Read the model definition and answer for the solid it produces. Units are mm, in the model's axes. Face numbers are marked on the shaded views. A direction names the side the tool comes from. Coordinates: 2 decimals unless noted, no trailing zeros. Write each loop counter-clockwise with the first axis right and the second up, starting at its lowest first coordinate (ties: lowest second). Pieces come first, ordered by that corner, then holes. Notation, with made-up numbers: (43, -38) -> (88, -38) arc R26 ccw to (88, -12) -> close; hole circle Ø1 at (20.5, 71.5). An arc over 180 degrees is marked (long way). Return JSON: item names as keys, results as strings.
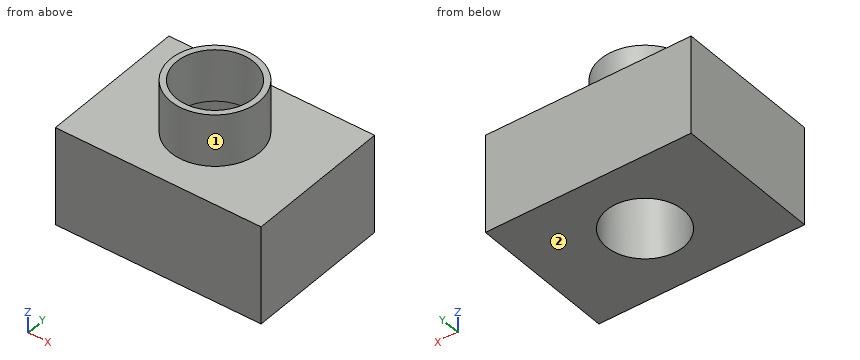
from build123d import *

# Parameters (mm, degrees)
F0_W      = 100.443094
F0_H      = 71.661144
F1_DEPTH  = 48.006
F2_R      = 21.614907
F2_R_2    = 18.770119
F3_DEPTH  = 25.4
F3_FACE_R = 18.770119
F4_DEPTH  = 86.36


with BuildPart() as f1:
    # F0 (on Top) → F1 (new body)
    with BuildSketch(Plane.XY):
        Rectangle(F0_W, F0_H)
    extrude(amount=F1_DEPTH)

    # F2 (on face) → F3 (join)
    with BuildSketch(Plane.XY.offset(48.006)):
        Circle(F2_R)
        Circle(F2_R_2, mode=Mode.SUBTRACT)
    extrude(amount=F3_DEPTH)

    # F3_face (on face) → F4 (cut)
    with BuildSketch(Plane.XY.offset(48.006)):
        Circle(F3_FACE_R)
    extrude(amount=-F4_DEPTH, mode=Mode.SUBTRACT)


solid = f1.part
1. The part is cut by section D-D (x = -28). Determine the outline of the cut face in (y, z).
Taken from the geometry:
{"outline": "(-35.83, 0) -> (35.83, 0) -> (35.83, 48.01) -> (-35.83, 48.01) -> close"}
2. The part is cut by section B-B (x = 0). Determine the outline of the cut face in (y, z).
Taken from the geometry:
{"outline": "(-35.83, 0) -> (-18.77, 0) -> (-18.77, 73.41) -> (-21.61, 73.41) -> (-21.61, 48.01) -> (-35.83, 48.01) -> close; (18.77, 0) -> (35.83, 0) -> (35.83, 48.01) -> (21.61, 48.01) -> (21.61, 73.41) -> (18.77, 73.41) -> close"}
3. The part is cut by section C-C (z = 8). Determine the outline of the cut face in (x, y).
Taken from the geometry:
{"outline": "(-50.22, -35.83) -> (50.22, -35.83) -> (50.22, 35.83) -> (-50.22, 35.83) -> close; hole circle Ø37.54 at (0, 0)"}
4. The part is cut by section A-A (y = 0). Determine the outline of the cut face in (x, z).
Taken from the geometry:
{"outline": "(-50.22, 0) -> (-18.77, 0) -> (-18.77, 73.41) -> (-21.61, 73.41) -> (-21.61, 48.01) -> (-50.22, 48.01) -> close; (18.77, 0) -> (50.22, 0) -> (50.22, 48.01) -> (21.61, 48.01) -> (21.61, 73.41) -> (18.77, 73.41) -> close"}
5. Consider L1, parallel to Y at x = 0, z = 37; L2, parallel to Y at x = 0, z = 56.75; L3, parallel to Z at x = -19.5, y = -11.5. Determine where each line is inside the solid, lowest interval first.
Taken from the geometry:
{"L1": "y = -35.83 to -18.77, 18.77 to 35.83", "L2": "y = -21.61 to -18.77, 18.77 to 21.61", "L3": "z = 0 to 48.01"}
6. A tool of negligible diameter and unlimited length cuts with its end or side. For the marked faces 1 and 2, from which of +Z, -Z, +X, -X, +Y, -Y can it reach the whole face along a straight path? Write none if from no direction.
Taken from the geometry:
{"face 1": "+Z", "face 2": "-Z, +X, -X, +Y, -Y"}
7. Flat-ended cylindrical pins translate along their axes: pin 1 Ø6 at (y, z) = (19.5, 53) entering from +X; pin 2 Ø12 at (x, y) = (-16.5, -24) entering from +Z. Find the tip coordinate at first contact, or state that the pin passes through.
Taken from the geometry:
{"pin 1": "stops at x = 13.96", "pin 2": "stops at z = 48.01"}
